The model under review builds one solid part; all positions refer to its coordinate system, in mm. Round coordinates to 2 decimals unless told otherwise and drop trailing zeros. Loops run counter-clockwise (first coordinate to the right, second up) from the corner with the lowest first, then second, coordinate; pieces in that order, holes last. Notation, with made-up numbers: (41, 4) -> (46, 4) arc R8 cw to (46, 14) -> close; hole circle Ø4 at (-5, 83). An arc over 180 degrees is marked (long way). Use a Markdown table: item, result. Add a question column.
1) Consider section B-B on z = 244. Give the boundary of the cut face in (x, y) (3 decimals).
2) Wall thickness on probe 1 along Z at (x, y) = (0.7, -1.5); probe 2 along Y at (x, z) = (2.35, 280.5); probe 3 along Z at (x, y) = (2.7, -15): over which ranges is each line inside the solid? List them lowest first.
3) Insertion check: pin 1 (1.5 mm diameter, centred on x = 1.5, y = -13, fed in from -Z); pin 2 (1 mm diameter, centred on x = 1, z = 126, fed in from -Y). Each pin has a flat end and moves straight along its axis. Give the tip position at first contact, or say it passes through.
4) Consider section A-A on x = 2.45. Give the boundary of the cut face in (y, z) (3 decimals).
5) Consider section C-C on y = -13. Give the boundary of the cut face in (x, z) (3 decimals), plus the area to 3 significant figures.
from build123d import *

# Parameters (mm, degrees)
SKETCH1_R           = 2.032
BOSS_EXTRUDE1_DEPTH = 3.175


with BuildPart() as part:
    # Sketch1 → Boss-Extrude1 (new body)
    # profile 1 of 3: a face of its own
    with BuildSketch(Plane(origin=(0, 0, 0), x_dir=(0, 0, -1), z_dir=(1, 0, 0))):
        with BuildLine():
            Line((47.169090512, -19.900738686), (3.175, 5.499261314))
            ThreePointArc((3.175, 5.499261314), (6.133628997, -1.643500936), (0, -6.35))
            Line((0, -6.35), (-1.701477372, -6.35))
            Line((-1.701477372, -6.35), (40.819090512, -30.899261314))
            ThreePointArc((40.819090512, -30.899261314), (49.493351826, -28.575), (47.169090512, -19.900738686))
        make_face()
        with Locations((43.994090512, -25.4)):
            Circle(SKETCH1_R, mode=Mode.SUBTRACT)
    # profile 2 of 3: a face of its own
    with BuildSketch(Plane(origin=(0, 0, 0), x_dir=(0, 0, -1), z_dir=(1, 0, 0))):
        with BuildLine():
            ThreePointArc((0, -6.35), (6.133628997, -1.643500936), (3.175, 5.499261314))
            ThreePointArc((3.175, 5.499261314), (1.643500936, 6.133628997), (0, 6.35))
            ThreePointArc((0, 6.35), (-6.133628997, 1.643500936), (-3.175, -5.499261314))
            Line((-3.175, -5.499261314), (-1.701477372, -6.35))
            Line((-1.701477372, -6.35), (0, -6.35))
        make_face()
        Circle(SKETCH1_R, mode=Mode.SUBTRACT)
    # profile 3 of 3: a face of its own
    with BuildSketch(Plane(origin=(0, 0, 0), x_dir=(0, 0, -1), z_dir=(1, 0, 0))):
        with BuildLine():
            ThreePointArc((-3.175, -5.499261314), (-6.133628997, 1.643500936), (0, 6.35))
            Line((0, 6.35), (-304.8, 6.35))
            ThreePointArc((-304.8, 6.35), (-311.15, 0), (-304.8, -6.35))
            Line((-304.8, -6.35), (-1.701477372, -6.35))
            Line((-1.701477372, -6.35), (-3.175, -5.499261314))
        make_face()
        with Locations((-304.8, 0)):
            Circle(SKETCH1_R, mode=Mode.SUBTRACT)
    extrude(amount=BOSS_EXTRUDE1_DEPTH)


solid = part.part
Result set:
| question | item | result |
|---|---|---|
| 1 | outline | (0, -6.35) -> (3.175, -6.35) -> (3.175, 6.35) -> (0, 6.35) -> close |
| 2 | probe 1 | -15.3 to -1.37, 1.37 to 303.43, 306.17 to 310.97 |
| 2 | probe 2 | -6.35 to 6.35 |
| 2 | probe 3 | -38.68 to -13.28 |
| 3 | pin 1 | z = -36.52 |
| 3 | pin 2 | y = -6.35 |
| 4 | outline | (-30.899, -40.819) arc R6.35 ccw to (-19.901, -47.169) -> (5.499, -3.175) arc R6.35 ccw to (6.35, 0) -> (6.35, 304.8) arc R6.35 ccw to (-6.35, 304.8) -> (-6.35, 1.701) -> close; hole circle Ø4.064 at (-25.4, -43.994); hole circle Ø4.064 at (0, 0); hole circle Ø4.064 at (0, 304.8) |
| 5 | outline | (0, -35.217) -> (3.175, -35.217) -> (3.175, -9.817) -> (0, -9.817) -> close |
| 5 | area | 80.6 mm2 |
